The model under review builds one solid part; all positions refer to its coordinate system, in mm. Round coordinates to 2 decimals unless told otherwise and drop trailing zeros. Order: outer loops, then holes, each group sorted by start corner. A loop starts at its lowest first (then second) coordinate and runs counter-clockwise, first axis right, second up. Notation, with made-up numbers: (39, 85) -> (71, 85) arc R37 ccw to (71, 124) -> close; hole circle Ø1 at (76.5, 24.25). An arc over 180 degrees is marked (long way). Use a Markdown table: item, result. Add a question column.
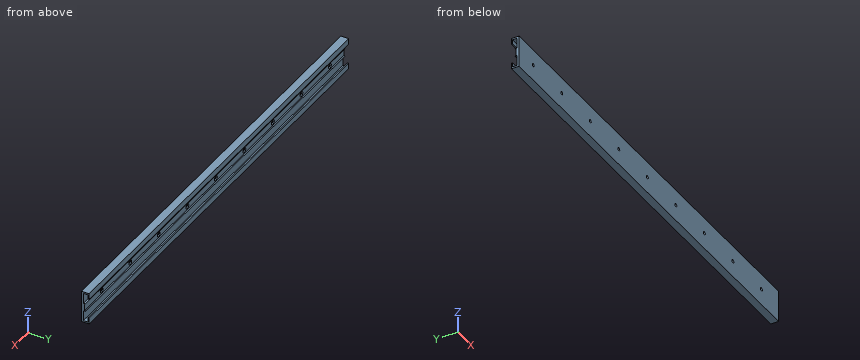
Autodesk Inventor part; units mm, degrees
ref_plane "YZ Plane" through (0, 0, 0) normal (1, 0, 0) x (0, 1, 0)
ref_plane "XZ Plane" through (0, 0, 0) normal (0, 1, 0) x (-1, 0, 0)
ref_plane "XY Plane" through (0, 0, 0) normal (0, 0, 1) x (1, 0, 0)
sketch "Sketch1" plane through (0, 0, 0) normal (1, 0, 0) x (0, 1, 0)
  line L0 (0, 0) -> (0, -40.005)
  line L1 (0, -40.005) -> (9.4996, -40.005)
  line L2 (0, 0) -> (9.4996, 0)
  line L3 (9.4996, 0) -> (9.4996, -7.493)
  line L4 (9.4996, 0) -> (16.9926, 0) construction
  line L5 (9.4996, -40.005) -> (9.4996, -32.512)
  line L6 (9.4996, -40.005) -> (16.9926, -40.005) construction
  line L7 (9.4996, -7.493) -> (8.001, -7.493)
  line L8 (9.4996, -32.512) -> (8.001, -32.512)
  line L9 (9.4996, -32.512) -> (10.9982, -32.512) construction
  line L10 (8.001, -7.493) -> (8.001, -2.0066)
  line L11 (8.001, -7.493) -> (13.4874, -7.493) construction
  line L12 (8.001, -32.512) -> (8.001, -37.9984)
  line L13 (8.001, -32.512) -> (13.4874, -32.512) construction
  line L14 (8.001, -2.0066) -> (2.4892, -2.0066)
  line L15 (2.4892, -2.0066) -> (2.4892, -15.0114)
  line L16 (2.4892, -15.0114) -> (4.9784, -15.0114)
  line L17 (8.001, -37.9984) -> (2.4892, -37.9984)
  line L18 (8.001, -37.9984) -> (13.5128, -37.9984) construction
  line L19 (2.4892, -37.9984) -> (2.4892, -24.9936)
  line L20 (2.4892, -24.9936) -> (4.9784, -24.9936)
  line L21 (4.9784, -15.0114) -> (3.9878, -15.0114) construction
  line L22 (3.9878, -15.0114) -> (3.9878, -24.9936) construction
  line L23 (4.9784, -15.0114) -> (3.9878, -16.002)
  line L24 (4.9784, -15.0114) -> (6.3793, -15.0114) construction
  line L25 (4.9784, -24.9936) -> (3.9878, -24.003)
  line L26 (4.9784, -24.9936) -> (6.3793, -24.9936) construction
  line L27 (3.9878, -24.003) -> (3.9878, -16.002)
  dimension "d0" = 40.005
  dimension "d1" = 9.4996
  dimension "d2" = 9.4996
  dimension "d3" = 7.493
  dimension "d4" = 90
  dimension "d5" = 7.493
  dimension "d6" = 90
  dimension "d7" = 1.4986
  dimension "d8" = 1.4986
  dimension "d9" = 180
  dimension "d10" = 5.4864
  dimension "d11" = 90
  dimension "d12" = 5.4864
  dimension "d13" = 90
  dimension "d22" = 5.5118
  dimension "d23" = 13.0048
  dimension "d24" = 2.4892
  dimension "d25" = 90
  dimension "d26" = 5.5118
  dimension "d27" = 180
  dimension "d28" = 13.0048
  dimension "d29" = 90
  dimension "d30" = 2.4892
  dimension "d31" = 90
  dimension "d32" = 0.9906
  dimension "d33" = 135
  dimension "d34" = 135
extrude "Extrusion1" add sketch "Sketch1" along normal blind 546.1
sketch "Sketch2" plane through (0, 3.9878, -16.002) normal (0, 1, 0) x (1, 0, 0)
  line L0 (0, 8.001) -> (0, 0)
  line L1 (0, 0) -> (546.1, 0)
  line L2 (546.1, 8.001) -> (546.1, 0)
  line L3 (0, 8.001) -> (546.1, 8.001)
  point P0 (0, -16.002)
  point P1 (29.9974, 3.9878)
  dimension "d37" = 29.9974
  dimension "d38" = 3.9878
hole "Hole1" at (29.9974, 3.9878, -19.9898) direction (0, -1, 0) diameter 3.9878 end through all countersink diameter 5.9944 countersink angle 82
pattern_linear "Rectangular Pattern1" count 9 spacing 59.9948 along (1, 0, 0) of "Hole1"
properties part number "aluminum slider"
Q1. To check wall thickness, follow line 1 along Z through (x, y) = (463, 3) (3 decimals); line 2 along Z through (x, y) = (231, 4.5) (3 decimals); line 3 along Y through (x, z) = (159, -5.5). State the ranges of each line that lie inside material, in increasing order.
Q2. For pin 1 (6.5 mm diameter, centred on x = 449.96, z = -19.99, fed in from -Y); pin 2 (3.5 mm diameter, centred on x = 149.99, z = -19.99, fed in from -Y); pin 3 (6.5 mm diameter, centred on x = 150, z = -20.5, fed in from +Y); pin 4 (5 mm diameter, centred on x = 30, z = -19.99, fed in from +Y), all flat-tipped, find the tip position at first contact; note any pin that passes through.
Q3. Add section A-A, the plane x = 46.5. Give the boundary of the cut face in (y, z) (3 decimals), then the cut area to 3 significant figures.
Return value:
| question | item | result |
|---|---|---|
| 1 | line 1 | -40.005 to -37.998, -24.994 to -15.011, -2.007 to 0 |
| 1 | line 2 | -40.005 to -37.998, -24.994 to -24.515, -15.49 to -15.011, -2.007 to 0 |
| 1 | line 3 | 0 to 2.49, 8 to 9.5 |
| 2 | pin 1 | y = 0 |
| 2 | pin 2 | through |
| 2 | pin 3 | y = 3.99 |
| 2 | pin 4 | y = 3.42 |
| 3 | outline | (0, -40.005) -> (9.5, -40.005) -> (9.5, -32.512) -> (8.001, -32.512) -> (8.001, -37.998) -> (2.489, -37.998) -> (2.489, -24.994) -> (4.978, -24.994) -> (3.988, -24.003) -> (3.988, -16.002) -> (4.978, -15.011) -> (2.489, -15.011) -> (2.489, -2.007) -> (8.001, -2.007) -> (8.001, -7.493) -> (9.5, -7.493) -> (9.5, 0) -> (0, 0) -> close |
| 3 | area | 160 mm² |
